Geometry check sheet. Reference: the model listing, model coordinates, mm. A direction names the side the tool comes from. Round coordinates to 2 decimals unless told otherwise and drop trailing zeros. Write each loop counter-clockwise with the first axis right and the second up, starting at its lowest first coordinate (ties: lowest second). Pieces come first, ordered by that corner, then holes. Notation, with made-up numbers: (81, 19) - (120, 19) arc R18 cw to (120, 32) - close; hole circle Ø4 at (-26.5, -35). An arc over 180 degrees is marked (long way). Return JSON: item names as keys, results as strings.
Autodesk Inventor part; units mm, degrees
ref_plane "YZ Plane" through (0, 0, 0) normal (1, 0, 0) x (0, 1, 0)
ref_plane "XZ Plane" through (0, 0, 0) normal (0, 1, 0) x (-1, 0, 0)
ref_plane "XY Plane" through (0, 0, 0) normal (0, 0, 1) x (1, 0, 0)
sketch "Эскиз1" plane through (0, 0, 0) normal (0, 1, 0) x (-1, 0, 0)
  line L0 (0, 0) -> (-132, 0)
  line L1 (-132, -165.5) -> (0, -165.5)
  line L2 (0, -165.5) -> (0, -157.5)
  line L3 (0, -157.5) -> (-3, -157.5)
  line L4 (0, 0) -> (0, -8)
  line L5 (0, -8) -> (-3, -8)
  line L6 (-3, -8) -> (-3, -157.5)
  line L7 (-132, -165.5) -> (-132, -157.5)
  line L8 (-132, -157.5) -> (-129, -157.5)
  line L9 (-129, -157.5) -> (-129, -8)
  line L10 (-129, -8) -> (-132, -8)
  line L11 (-132, -8) -> (-132, 0)
  line L12 (-30.5, -100.75) -> (-101.5, -100.75)
  line L13 (-101.5, -100.75) -> (-101.5, -64.75)
  line L14 (-101.5, -64.75) -> (-30.5, -64.75)
  line L15 (-30.5, -64.75) -> (-30.5, -100.75)
  circle A0 centre (-59.8, -59) radius 3
  circle A1 centre (-72.2, -59) radius 3
  circle A2 centre (-85.5, -61.8) radius 1.5
  circle A3 centre (-93.5, -59) radius 1.5
  circle A4 centre (-93.5, -106.5) radius 1.5
  circle A5 centre (-85.5, -103.7) radius 1.5
  circle A6 centre (-72.2, -106.5) radius 3
  circle A7 centre (-59.8, -106.5) radius 3
  circle A8 centre (-46.5, -103.7) radius 1.5
  circle A9 centre (-38.5, -106.5) radius 1.5
  circle A10 centre (-38.5, -59) radius 1.5
  circle A11 centre (-46.5, -61.8) radius 1.5
  circle A12 centre (-10, -35) radius 1.5
  circle A13 centre (-10, -51) radius 1.5
  circle A14 centre (-24, -51) radius 1.5
  circle A15 centre (-24, -35) radius 1.5
  circle A16 centre (-24, -114.5) radius 1.5
  circle A17 centre (-10, -114.5) radius 1.5
  circle A18 centre (-10, -130.5) radius 1.5
  circle A19 centre (-24, -130.5) radius 1.5
  circle A20 centre (-108, -130.5) radius 1.5
  circle A21 centre (-108, -114.5) radius 1.5
  circle A22 centre (-122, -114.5) radius 1.5
  circle A23 centre (-122, -130.5) radius 1.5
  circle A24 centre (-122, -51) radius 1.5
  circle A25 centre (-108, -51) radius 1.5
  circle A26 centre (-108, -35) radius 1.5
  circle A27 centre (-122, -35) radius 1.5
extrude "Выдавливание1" add sketch "Эскиз1" along normal blind 10
sketch "Эскиз2" plane through (0, 10, 0) normal (0, 1, 0) x (1, 0, 0)
  line L0 (132, 157.5) -> (132, 165.5)
  line L1 (0, 165.5) -> (0, 157.5)
  line L2 (0, 0) -> (132, 0)
  line L3 (132, 165.5) -> (0, 165.5)
  circle A0 centre (10, 114.5) radius 1.5
  circle A1 centre (10, 130.5) radius 1.5
  line L4 (10, 114.5) -> (10, 130.5)
  dimension "d59" = 132
  dimension "d60" = 165.5
properties part number "maze_01_test"
(1) Release check for a two-part mould opening along Z. For faces 5 (the face through (67, 5, -165.5)), 6 (the face through (0, 5, -162)), 7 (the face through (101.5, 5, -83)) record: pulls with the +Z half, pulls with the -Z half, needs draft (parallel to the pull), parting line crosses it, or undercut.
Response values:
{"face 5": "pulls with the -Z half", "face 6": "needs draft", "face 7": "undercut"}
(2) Section check A-A, the plane x = 72.2. Enter the section's corners in (y, z), plus the area to 4 significant figures.
Response values:
{"outline": "(0, -165.5) - (10, -165.5) - (10, -109.5) - (0, -109.5) - close; (0, -103.5) - (10, -103.5) - (10, -100.75) - (0, -100.75) - close; (0, -64.75) - (10, -64.75) - (10, -62) - (0, -62) - close; (0, -56) - (10, -56) - (10, 0) - (0, 0) - close", "area": "1,175 mm^2"}
(3) Section check B-B, the plane z = -94. Enter the section's corners in (x, y), plus the area to 3 significant figures.
Response values:
{"outline": "(3, 0) - (30.5, 0) - (30.5, 10) - (3, 10) - close; (101.5, 0) - (129, 0) - (129, 10) - (101.5, 10) - close", "area": "550 mm^2"}
(4) Access from +Z, -Z, +X, -X, +Y, -Y to the whole of each face (thin tool, end or side, straight path). Record for faces 1 (the face through (67, 10, -63)), 2 (the face through (129, 5, -84)), 3 (the face through (66, 5, -64.75)), 4 (the face through (3, 5, -82)).
Response values:
{"face 1": "+Z, -Z, +X, -X, +Y", "face 2": "+X, +Y, -Y", "face 3": "+Y, -Y", "face 4": "-X, +Y, -Y"}
(5) Section check D-D, the plane y = 7.25. Give the number of separate pieces and of enclosed holes in the cut face, plus the area to 3 significant figures.
Response values:
{"separate pieces": "1", "enclosed holes": "29", "area": "18,100 mm^2"}
(6) Material ranges on line 1 along Z through (x, y) = (108, 5); line 2 along Z through (x, y) = (72.2, 3); line 3 along X through (y, z) = (0.5, -106), recorded low to high. Write a range as [from, to].
Response values:
{"line 1": "z = [-165.5, -132], [-129, -116], [-113, -52.5], [-49.5, -36.5], [-33.5, 0]", "line 2": "z = [-165.5, -109.5], [-103.5, -100.75], [-64.75, -62], [-56, 0]", "line 3": "x = [3, 37.09], [39.91, 56.84], [62.76, 69.24], [75.16, 92.09], [94.91, 129]"}
(7) Gauge pin test, flat ends, axial feed: pin 1 (6 mm diameter, centred on y = 2, z = -117.5, fed in from -X); pin 2 (4 mm diameter, centred on x = 47, z = -147, fed in from -Y); pin 3 (1 mm diameter, centred on y = 8, z = -119, fed in from +X). Record the tip position at first contact, or that the pin passes through.
Response values:
{"pin 1": "stops at x = 3", "pin 2": "stops at y = 0", "pin 3": "stops at x = 129"}
(8) Section check C-C, the plane x = 52. Enter the section's corners in (y, z).
Response values:
{"outline": "(0, -165.5) - (10, -165.5) - (10, -100.75) - (0, -100.75) - close; (0, -64.75) - (10, -64.75) - (10, 0) - (0, 0) - close"}
